```python
from build123d import *

# Parameters (mm, degrees)
SKETCH1_R           = 2.2
BOSS_EXTRUDE1_DEPTH = 6


with BuildPart() as part:
    # Sketch1 → Boss-Extrude1 (new body)
    with BuildSketch(Plane.XY.offset(6)):
        Polygon((-54, 85), (-54, 115), (-116, 115), (-116, -115), (116, -115), (116, 115), (-14, 115), (-14, 85), align=None)
        with Locations(Location((-109.6, 62, 0), (0, 0, 180))):
            Circle(SKETCH1_R, mode=Mode.SUBTRACT)
        with Locations(Location((108.6, -62, 0), (0, 0, 180))):
            Circle(SKETCH1_R, mode=Mode.SUBTRACT)
        with Locations(Location((108.6, 62, 0), (0, 0, 180))):
            Circle(SKETCH1_R, mode=Mode.SUBTRACT)
        with Locations(Location((-109.6, -62, 0), (0, 0, 180))):
            Circle(SKETCH1_R, mode=Mode.SUBTRACT)
    extrude(amount=-BOSS_EXTRUDE1_DEPTH)


solid = part.part
```
For this review, take the finished solid that the model builds, in its own axes (mm). A direction names the side the tool comes from. Coordinates: 2 decimals unless noted, no trailing zeros. Write each loop counter-clockwise with the first axis right and the second up, starting at its lowest first coordinate (ties: lowest second). Pieces come first, ordered by that corner, then holes. Notation, with made-up numbers: (19.5, 64.25) - (35.5, 64.25) arc R10 cw to (35.5, 80.25) - close; hole circle Ø4 at (75.5, 64). An arc over 180 degrees is marked (long way). Put each result on its own line as item: value.
1. Mouldability with a two-part tool opening along X and no side actions: class faces 1 (the flat face through (-116, 2, 3)), 2 (the flat face through (-2, 2, 0)), 3 (the flat face through (-54, 100, 3)), 4 (the flat face through (-34, 85, 3)) as released by +X, released by -X, zero draft, split by the parting line, or undercut.
Values found:
face 1: released by -X
face 2: zero draft
face 3: undercut
face 4: undercut
2. For pin 1 (3.5 mm diameter, centred on x = 108.6, y = 62, fed in from +Z) (3 decimals); pin 2 (7 mm diameter, centred on x = -109.6, y = 62, fed in from +Z); pin 3 (1.8 mm diameter, centred on x = -25, z = 3.5, fed in from +Y), all flat-tipped, find the tip position at first contact; note any pin that passes through.
Values found:
pin 1: through
pin 2: z = 6
pin 3: y = 85
3. Wall thickness on probe 1 along X at (y, z) = (-62, 4.45); probe 2 along Y at (x, z) = (108.6, 3.9); probe 3 along X at (y, z) = (95, 2): over which ranges is each line inside the solid? List them lowest first.
Values found:
probe 1: -116 to -111.8, -107.4 to 106.4, 110.8 to 116
probe 2: -115 to -64.2, -59.8 to 59.8, 64.2 to 115
probe 3: -116 to -54, -14 to 116
4. Machinability: for faces 5 (the flat face through (116, -2, 3)), 6 (the flat face through (-14, 100, 3)), which of the approach directions +Z, -Z, +X, -X, +Y, -Y give a long, thin tool a straight path to every point of the face, cutting with its end or side? Answer none if there is none.
Values found:
face 5: +Z, -Z, +X, +Y, -Y
face 6: +Z, -Z, +Y
5. Add section A-A, the plane z = 1.35. Give the boundary of the cut face in (x, y).
Values found:
outline: (-116, -115) - (116, -115) - (116, 115) - (-14, 115) - (-14, 85) - (-54, 85) - (-54, 115) - (-116, 115) - close; hole circle Ø4.4 at (-109.6, -62); hole circle Ø4.4 at (-109.6, 62); hole circle Ø4.4 at (108.6, -62); hole circle Ø4.4 at (108.6, 62)
